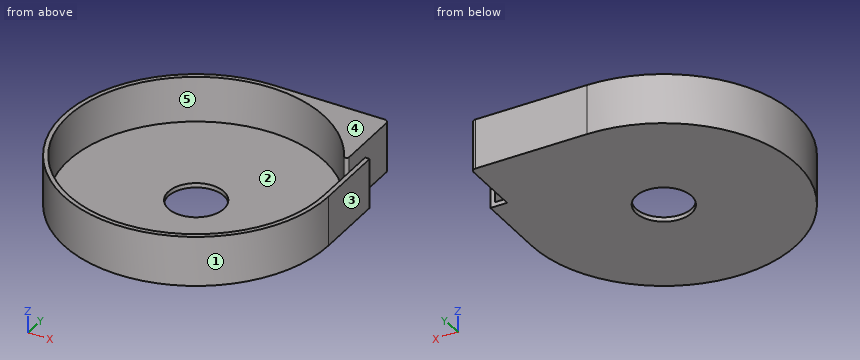
from build123d import *

# Parameters (mm, degrees)
SKETCH001_R  = 5
PAD_DEPTH    = 0.8
PAD001_DEPTH = 8.2


with BuildPart() as part:
    # Sketch001 → Pad (new body)
    with BuildSketch(Plane.XY):
        with BuildLine():
            ThreePointArc((0, 23.8), (-16.829141, -16.829141), (23.8, 0))
            Line((23.8, 12.662984), (23.8, 0))
            Line((20.8, 12.662984), (23.8, 12.662984))
            Line((20.8, 23), (20.8, 12.662984))
            ThreePointArc((20.8, 23), (20.565685, 23.565685), (20, 23.8))
            Line((0, 23.8), (20, 23.8))
        make_face()
        Circle(SKETCH001_R, mode=Mode.SUBTRACT)
    extrude(amount=PAD_DEPTH)

    # Sketch002 → Pad001 (join)
    with BuildSketch(Plane.XY.offset(0.8)):
        with BuildLine():
            ThreePointArc((0, 23.8), (-16.829141, -16.829141), (23.8, 0))
            Line((23.8, 0), (23.8, 12.662984))
            Line((23, 12.662984), (23.8, 12.662984))
            Line((23, 12.662984), (23, 0))
            ThreePointArc((20.051282, 11.267035), (-22.250612, -5.823251), (23, 0))
            ThreePointArc((20.051282, 11.267035), (20.501274, 11.076017), (20.8, 11.462984))
            Line((20.8, 23), (20.8, 11.462984))
            ThreePointArc((20.8, 23), (20.565685, 23.565685), (20, 23.8))
            Line((0, 23.8), (20, 23.8))
        make_face()
    extrude(amount=PAD001_DEPTH)


solid = part.part
Geometry: final body of the model. Coordinates: model frame, mm. Face numbers are marked on the shaded views. A direction names the side the tool comes from. Give positions to 0.01 mm unless a question says otherwise; leave off trailing zeros. Write each loop counter-clockwise with the first axis right and the second up, starting at its lowest first coordinate (ties: lowest second). Pieces come first, ordered by that corner, then holes. Notation, with made-up numbers: M -7,-27.75 L 39,-27.75 A4 ccw 39,-23.75 Z; hole C -37.75,12 d2. An arc over 180 degrees is marked long. Answer in a Markdown table with one row per item. Add a question column.
(1) Section A-A on x = 3. Return loops of the section in (y, z), and give its area (3 significant figures).
(2) First-contact query: pin 1 (4 mm diameter, centred on x = -3, z = 1.5, fed in from -Y); pin 2 (4.5 mm diameter, centred on y = 15, z = 3, fed in from +X); pin 3 (13 mm diameter, centred on x = 0, y = 0, fed in from +Z). Flat tips, straight axial feed; report the tip coordinate or a pass-through.
(3) Reachability of the marked faces 4 and 5 from +Z, -Z, +X, -X, +Y, -Y: full face, straight path, thin tool, end or side. Return the list, or none.
(4) Section B-B on y = -8. Return loops of the section in (x, z).
(5) Ray query, line 1 (X direction, y = -0.5, z = 7); line 2 (Z direction, x = -1.5, y = 14); line 3 (Y direction, x = -5, z = 1.5). Return the intervals inside material, ascending.
(6) Mould query, pull axis Y, two halves, no side actions, for the marked faces 1, 2 and 3. Classes: +Y half, -Y half, draft (parallel to the pull), parting line (faces both ways), or undercut.
(7) Section C-C on z = 2. Return loops of the section in (x, y).
Result set:
| question | item | result |
|---|---|---|
| 1 | outline | M -23.61,0 L -4,0 L -4,0.8 L -22.8,0.8 L -22.8,9 L -23.61,9 Z; M 4,0 L 23.8,0 L 23.8,9 L 22.8,9 L 22.8,0.8 L 4,0.8 Z |
| 1 | area | 46.3 mm^2 |
| 2 | pin 1 | stops at y = -23.78 |
| 2 | pin 2 | stops at x = 20.8 |
| 2 | pin 3 | stops at z = 0.8 |
| 3 | face 4 | +Z, +X, -X, +Y, -Y |
| 3 | face 5 | +Z |
| 4 | outline | M -22.42,0 L 22.42,0 L 22.42,9 L 21.56,9 L 21.56,0.8 L -21.56,0.8 L -21.56,9 L -22.42,9 Z |
| 5 | line 1 | x = -23.79 to -22.99, 22.99 to 23.79 |
| 5 | line 2 | z = 0 to 0.8 |
| 5 | line 3 | y = -23.27 to -22.45, 22.45 to 23.27 |
| 6 | face 1 | parting line |
| 6 | face 2 | undercut |
| 6 | face 3 | draft |
| 7 | outline | M 0,23.8 A23.8 ccw long 23.8,0 L 23.8,12.66 L 23,12.66 L 23,0 A23 cw long 20.05,11.27 A0.4 ccw 20.8,11.46 L 20.8,23 A0.8 ccw 20,23.8 Z |
